Read the model definition and answer for the solid it produces. Units are mm, in the model's axes. Face numbers are marked on the shaded views. A direction names the side the tool comes from. Coordinates: 2 decimals unless noted, no trailing zeros. Write each loop counter-clockwise with the first axis right and the second up, starting at its lowest first coordinate (ties: lowest second). Pieces come first, ordered by that corner, then holes. Notation, with made-up numbers: (79.25, -14.75) - (89.25, -14.75) arc R25 ccw to (89.25, -2.75) - close; hole circle Ø6 at (-21.5, 79). An arc over 180 degrees is marked (long way). Use a Markdown table: item, result.
from build123d import *

# Parameters (mm, degrees)
BOSS_EXTRUDE1_DEPTH = 13.8
CUT_EXTRUDE1_DEPTH  = 8.3
SKETCH5_R           = 0.75
CUT_EXTRUDE3_DEPTH  = 4.5
SKETCH7_RX          = 5
SKETCH7_RY          = 3.3
BOSS_EXTRUDE5_DEPTH = 1.6
FILLET1_R           = 1
CUT_EXTRUDE4_DEPTH  = 8.3


with BuildPart() as part:
    # Sketch1 → Boss-Extrude1 (new body)
    with BuildSketch(Plane.XY):
        with BuildLine():
            Line((1.58113883, -2.25), (3.605551275, -2.25))
            ThreePointArc((3.605551275, -2.25), (4.25, 0), (3.605551275, 2.25))
            Line((3.605551275, 2.25), (1.58113883, 2.25))
            ThreePointArc((1.58113883, 2.25), (-2.75, 0), (1.58113883, -2.25))
        make_face()
    extrude(amount=BOSS_EXTRUDE1_DEPTH)

    # Sketch3 → Cut-Extrude1 (cut)
    with BuildSketch(Plane.XY.offset(13.8)):
        with BuildLine():
            Line((1, -1.118033989), (1, 1.118033989))
            ThreePointArc((1, 1.118033989), (-1.5, 0), (1, -1.118033989))
        make_face()
    extrude(amount=-CUT_EXTRUDE1_DEPTH, mode=Mode.SUBTRACT)

    # Sketch5 → Cut-Extrude3 (cut)
    with BuildSketch(Plane(origin=(4.25, 0, 0), x_dir=(0, 0, -1), z_dir=(1, 0, 0))):
        with Locations((-11.3, 0)):
            Circle(SKETCH5_R)
        with Locations((-7.3, 0)):
            Circle(SKETCH5_R)
    extrude(amount=-CUT_EXTRUDE3_DEPTH, mode=Mode.SUBTRACT)

    # Sketch7 → Boss-Extrude5 (add)
    with BuildSketch(Plane(origin=(0, 0, 0), x_dir=(-1, 0, 0), z_dir=(0, 0, -1))):
        with Locations(Location((0, 0), (0, 0, 0))):
            Ellipse(SKETCH7_RX, SKETCH7_RY)
    extrude(amount=BOSS_EXTRUDE5_DEPTH)

    # Fillet1
    fillet1_edges = [part.edges().sort_by_distance(p)[0] for p in [
        (3.605551275, -2.25, 6.9),
        (3.605551275, 2.25, 6.9),
    ]]
    fillet(fillet1_edges, radius=FILLET1_R)

    # Sketch8 → Cut-Extrude4 (cut)
    with BuildSketch(Plane.XY.offset(13.8)):
        with BuildLine():
            Line((1.06, 1.144552314), (1.06, -1.144552314))
            ThreePointArc((1.06, -1.144552314), (-1.56, 0), (1.06, 1.144552314))
        make_face()
        with BuildLine():
            Line((1, 1.118033989), (1, -1.118033989))
            ThreePointArc((1, -1.118033989), (-1.5, 0), (1, 1.118033989))
        make_face(mode=Mode.SUBTRACT)
    extrude(amount=-CUT_EXTRUDE4_DEPTH, mode=Mode.SUBTRACT)


solid = part.part
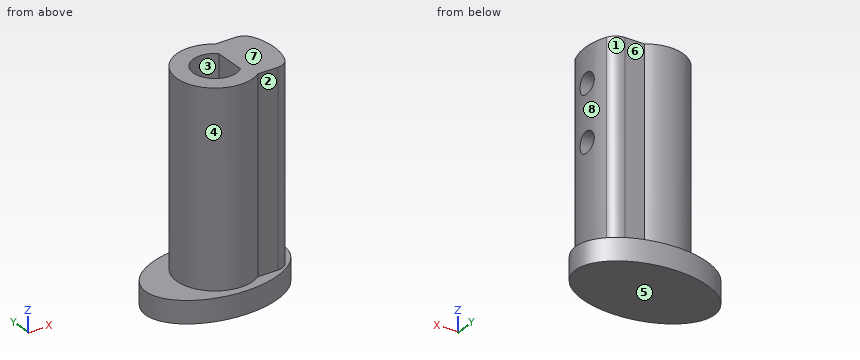
(1) A cutting plane is placed at B-B, the plane y = 0. Count the separate pieces of the cut face and the enclosed holes in it, and give its area (3 significant figures).
Report:
| item | result |
|---|---|
| separate pieces | 3 |
| enclosed holes | 0 |
| area | 81.3 mm² |
(2) A cutting plane is placed at C-C, the plane z = 4.75. Write down the section's boundary in (x, y).
Report:
| item | result |
|---|---|
| outline | (1.58, -2.25) - (3, -2.25) arc R1 ccw to (3.92, -1.63) arc R4.25 ccw to (3.92, 1.63) arc R1 ccw to (3, 2.25) - (1.58, 2.25) arc R2.75 ccw (long way) to start |
(3) A cutting plane is placed at D-D, the plane z = 11. Write down the section's boundary in (x, y), and give its area (3 significant figures).
Report:
| item | result |
|---|---|
| outline | (1.06, -1.14) arc R1.56 cw (long way) to (1.06, 1.14) - (1.06, 0.69) - (4.19, 0.69) arc R4.25 ccw to (3.92, 1.63) arc R1 ccw to (3, 2.25) - (1.58, 2.25) arc R2.75 ccw (long way) to (1.58, -2.25) - (3, -2.25) arc R1 ccw to (3.92, -1.63) arc R4.25 ccw to (4.19, -0.69) - (1.06, -0.69) - close |
| area | 19.8 mm² |
(4) Straight lines are drawn through the part: L1, parallel to Z at x = 2.35, y = 0; L2, parallel to Z at x = -3, y = 2; L3, parallel to Y at x = 3.3, z = 11.3. For each, find the intervals that lie inside material, in ascending order.
Report:
| item | result |
|---|---|
| L1 | z = -1.6 to 6.55, 8.05 to 10.55, 12.05 to 13.8 |
| L2 | z = -1.6 to 0 |
| L3 | y = -2.2 to -0.75, 0.75 to 2.2 |
(5) A cutting plane is placed at A-A, the plane z = 9. Write down the section's boundary in (x, y), and give its area (3 significant figures).
Report:
| item | result |
|---|---|
| outline | (1.58, -2.25) - (3, -2.25) arc R1 ccw to (3.92, -1.63) arc R4.25 ccw to (3.92, 1.63) arc R1 ccw to (3, 2.25) - (1.58, 2.25) arc R2.75 ccw (long way) to start; hole (1.06, -1.14) - (1.06, 1.14) arc R1.56 ccw (long way) to start |
| area | 24.2 mm² |
(6) For the marked faces 4, 5, 6, 7 and 8, determine the directions among +Z, -Z, +X, -X, +Y, -Y from which every point of the face is accessible in a straight line to the end or side of a thin tool.
Report:
| item | result |
|---|---|
| face 4 | +Z |
| face 5 | -Z, +X, -X, +Y, -Y |
| face 6 | +Z, +X, +Y |
| face 7 | +Z, +X, -X, +Y, -Y |
| face 8 | +Z, +X |
(7) The mould has two halves that part along Y. Classify the marked faces 1, 2 and 3: pulls with the +Y half, pulls with the -Y half, needs draft (parallel to the pull), parting line crosses it, or undercut.
Report:
| item | result |
|---|---|
| face 1 | pulls with the +Y half |
| face 2 | pulls with the -Y half |
| face 3 | undercut |
(8) Each of these flat-tipped pins is pushed along its axis until it touches: P1, Ø2.5, axis at y = 0, z = 11.3, coming from the +X side; P2, Ø1.5, axis at x = -3, z = 12, coming from the +Y side; P3, Ø1.5, axis at y = 2, z = 11.5, coming from the -X side. Where does it stop, or does it pass through?
Report:
| item | result |
|---|---|
| P1 | stops at x = 4.25 |
| P2 | stops at y = 1.58 |
| P3 | stops at x = -2.45 |
